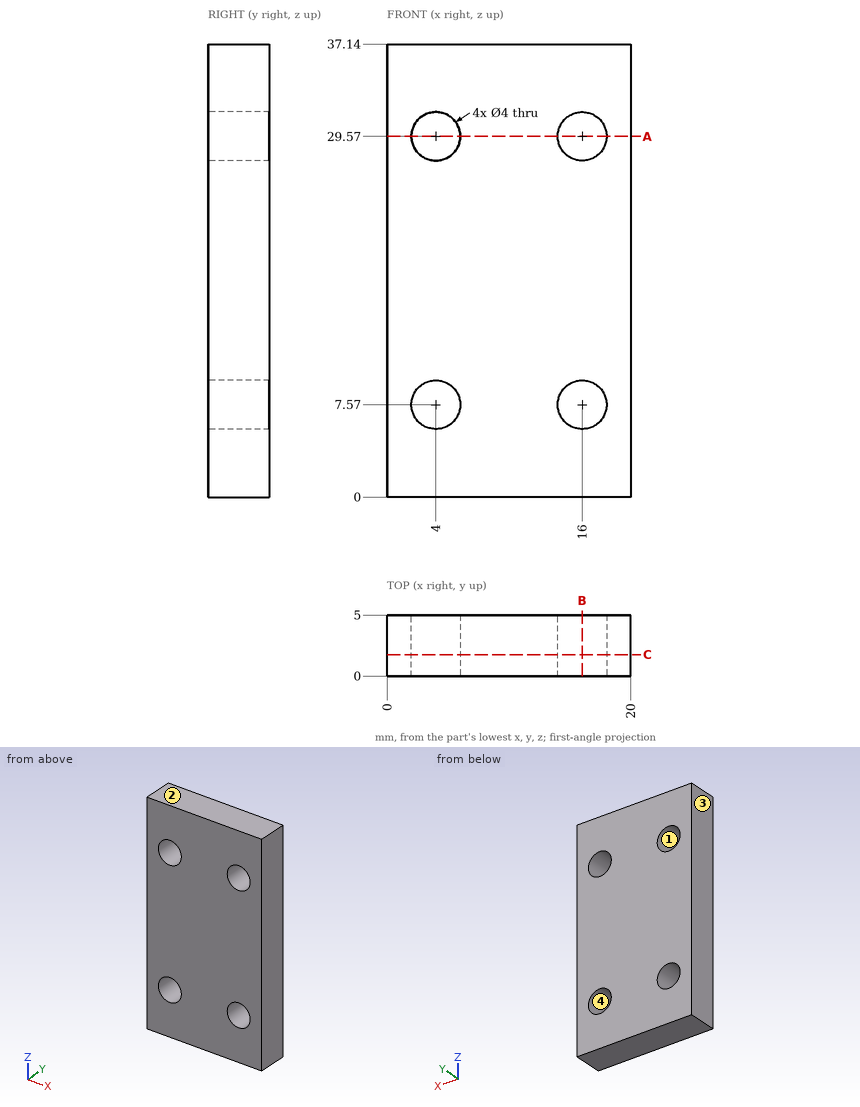
Geometry: see drawing. Coordinates: mm, zero at the bounding-box minimum. Round coordinates to 2 decimals unless told otherwise and drop trailing zeros. Write each loop counter-clockwise with the first axis right and the second up, starting at its lowest first coordinate (ties: lowest second). Pieces come first, ordered by that corner, then holes.
1) Cut plane C-C (y = 1.75). Return the cut outline in (x, z).
2) Cut plane B-B (x = 16). Return the cut outline in (y, z), then the cut area to 3 significant figures.
3) Cut plane A-A (z = 29.57). Return the cut outline in (x, y), then the cut area to 3 significant figures.
4) Contact query for flat-ended pins moving along their axis: P1, Ø1.5, axis at x = 11, z = 15, coming from the -Y side; P2, Ø2.5, axis at x = 16, z = 29.57, coming from the +Y side. Output: stop coordinate, or through.
5) Draft query along Z for the marked faces 1, 2, 3 and 4. Return one class per face: pulls with the +Z half, pulls with the -Z half, needs draft (parallel to the pull), parting line crosses it, or undercut.
6) Ray query, L1, parallel to Z at x = 4, y = 2; L2, parallel to Z at x = 2.5, y = 0.5. Return the intervals inside material, ascending.
Geometry says:
1. outline: (0, 0) - (20, 0) - (20, 37.14) - (0, 37.14) - close; hole circle Ø4 at (4, 7.57); hole circle Ø4 at (4, 29.57); hole circle Ø4 at (16, 7.57); hole circle Ø4 at (16, 29.57)
2. outline: (0, 0) - (5, 0) - (5, 5.57) - (0, 5.57) - close; (0, 9.57) - (5, 9.57) - (5, 27.57) - (0, 27.57) - close; (0, 31.57) - (5, 31.57) - (5, 37.14) - (0, 37.14) - close
2. area: 146 mm2
3. outline: (0, 0) - (2, 0) - (2, 5) - (0, 5) - close; (6, 0) - (14, 0) - (14, 5) - (6, 5) - close; (18, 0) - (20, 0) - (20, 5) - (18, 5) - close
3. area: 60.0 mm2
4. P1: stops at y = 0
4. P2: passes through
5. face 1: undercut
5. face 2: pulls with the +Z half
5. face 3: needs draft
5. face 4: undercut
6. L1: z = 0 to 5.57, 9.57 to 27.57, 31.57 to 37.14
6. L2: z = 0 to 6.25, 8.89 to 28.25, 30.89 to 37.14
